```python
from build123d import *
from build123d.topology import SkipClean

# Parameters (mm, degrees)
BOSS_EXTRUDE1_START = 92.075
SKETCH1_R           = 139.7
BOSS_EXTRUDE1_DEPTH = 6.35
BOSS_EXTRUDE2_START = -92.075
SKETCH2_R           = 139.7
BOSS_EXTRUDE2_DEPTH = 12.7
BOSS_EXTRUDE3_START = 165.1
BOSS_EXTRUDE3_DEPTH = 165.1
CIRPATTERN1_COUNT   = 6
SKETCH8_R           = 38.1
BOSS_EXTRUDE4_DEPTH = 63.5
SKETCH9_R           = 19.05
CUT_EXTRUDE1_DEPTH  = 76.2
SKETCH10_R          = 101.6
CUT_EXTRUDE2_DEPTH  = 6.35


with BuildPart() as part:
    # Sketch1 → Boss-Extrude1 (new body)
    with BuildSketch(Plane(origin=(0, 0, 0), x_dir=(1, 0, 0), z_dir=(0, 1, 0)).offset(BOSS_EXTRUDE1_START)):
        with Locations(Location((0, 0, 0), (0, 0, 270))):
            Circle(SKETCH1_R)
    extrude(amount=-BOSS_EXTRUDE1_DEPTH)



with BuildPart() as body_2:
    # Sketch2 → Boss-Extrude2 (new body)
    with BuildSketch(Plane(origin=(0, 0, 0), x_dir=(1, 0, 0), z_dir=(0, 1, 0)).offset(BOSS_EXTRUDE2_START)):
        with Locations(Location((0, 0, 0), (0, 0, 270))):
            Circle(SKETCH2_R)
    extrude(amount=BOSS_EXTRUDE2_DEPTH)


with BuildPart() as part_1:
    add(part.part)

    add(body_2.part)  # Boss-Extrude3 merges body 2
    # Sketch3 → Boss-Extrude3 (add)
    with BuildSketch(Plane(origin=(0, -79.375, 0), x_dir=(1, 0, 0), z_dir=(0, 1, 0)).offset(BOSS_EXTRUDE3_START)):
        with BuildLine():
            Line((122.269799969, -59.297454545), (125.697925202, -60.96))
            ThreePointArc((125.697925202, -60.96), (135.408353278, -34.360847815), (139.555607197, -6.35))
            Line((139.555607197, -6.35), (139.555607197, 0))
            Line((139.555607197, 0), (76.563607197, 0))
            Line((76.563607197, 0), (76.563607197, -6.35))
            Line((76.563607197, -6.35), (135.741554433, -6.35))
            ThreePointArc((135.741554433, -6.35), (131.694050685, -33.507747077), (122.269799969, -59.297454545))
        make_face()
    boss_extrude3 = extrude(amount=-BOSS_EXTRUDE3_DEPTH)

    # CirPattern1: Boss-Extrude3 ×6 about axis
    with SkipClean():  # the faces are left unmerged after this step: merging them gives an invalid solid
        cirpattern1_axis = Axis((0, 0, 0), (0, 1, 0))
        for i in range(1, CIRPATTERN1_COUNT):
            add(boss_extrude3.rotate(cirpattern1_axis, i * 360 / CIRPATTERN1_COUNT))

    # Sketch8 → Boss-Extrude4 (add)
    with SkipClean():  # the faces are left unmerged after this step: merging them gives an invalid solid
        with BuildSketch(Plane.XZ.offset(92.075)):
            with Locations(Location((0, 0, 0), (0, 0, 270))):
                Circle(SKETCH8_R)
        extrude(amount=BOSS_EXTRUDE4_DEPTH)

    # Sketch9 → Cut-Extrude1 (cut)
    with SkipClean():  # the faces are left unmerged after this step: merging them gives an invalid solid
        with BuildSketch(Plane.XZ.offset(155.575)):
            with Locations(Location((0, 0, 0), (0, 0, 270))):
                Circle(SKETCH9_R)
        extrude(amount=-CUT_EXTRUDE1_DEPTH, mode=Mode.SUBTRACT)

    # Sketch10 → Cut-Extrude2 (cut)
    with SkipClean():  # the faces are left unmerged after this step: merging them gives an invalid solid
        with BuildSketch(Plane(origin=(0, 92.075, 0), x_dir=(1, 0, 0), z_dir=(0, 1, 0))):
            with Locations(Location((0, 0, 0), (0, 0, 270))):
                Circle(SKETCH10_R)
        extrude(amount=-CUT_EXTRUDE2_DEPTH, mode=Mode.SUBTRACT)


solid = part_1.part
```
Design review of the part built by this model. Coordinates are the model's own, in mm. A direction names the side the tool comes from. Give positions to 0.01 mm unless a question says otherwise; leave off trailing zeros. Loops run counter-clockwise (first coordinate to the right, second up) from the corner with the lowest first, then second, coordinate; pieces in that order, holes last. Notation, with made-up numbers: (-15.75, -2.5) -> (20.25, -2.5) arc R29 ccw to (20.25, 35.5) -> close; hole circle Ø2 at (55.5, 20.5). An arc over 180 degrees is marked (long way). One line per item, written item: value.
Q1. For L1, parallel to X at y = 88.75, z = 0; L2, parallel to Z at x = -45.5, y = -71, list the stretches that pass through material, from the lowest coordinate up.
Numbers:
L1: x = -139.7 to -101.6, 101.6 to 139.7
L2: z = -132.08 to -128.05, -91.51 to -78.81, 66.11 to 78.81
Q2. Draft analysis for pull direction Z (two halves, no side actions). For faces 4 (the flat face through (-103, 92.075, 10)), 5 (the flat face through (-109, 4, 0)), state which applies: pulls with the +Z half, pulls with the -Z half, needs draft (parallel to the pull), parting line crosses it, or undercut.
Numbers:
face 4: needs draft
face 5: undercut
Q3. Machinability: for faces 1 (the flat face through (-5, 85.725, 113)), 2 (the cylindrical face through (-131.79, 4.33, -33.13)), 3 (the flat face through (106, 4, 6.35)), which of the approach directions +Z, -Z, +X, -X, +Y, -Y give a long, thin tool a straight path to every point of the face, cutting with its end or side? Answer none if there is none.
Numbers:
face 1: none
face 2: +X
face 3: -X
Q4. We need section A-A on x = 0. Give the boundary of the cut face in (y, z) (3 decimals).
Numbers:
outline: (-155.575, -38.1) -> (-92.075, -38.1) -> (-92.075, -139.7) -> (-79.375, -139.7) -> (-79.375, -19.05) -> (-155.575, -19.05) -> close; (-155.575, 19.05) -> (-79.375, 19.05) -> (-79.375, 139.7) -> (-92.075, 139.7) -> (-92.075, 38.1) -> (-155.575, 38.1) -> close; (85.725, -139.7) -> (92.075, -139.7) -> (92.075, -101.6) -> (85.725, -101.6) -> close; (85.725, 101.6) -> (92.075, 101.6) -> (92.075, 139.7) -> (85.725, 139.7) -> close
Q5. We need section D-D on y = -97.5. Give the boundary of the cut face in (x, z).
Numbers:
outline: circle Ø76.2 at (0, 0); hole circle Ø38.1 at (0, 0)
Q6. For pin 1 Ø8 at (x, y) = (12, 24) entering from -Z; pin 2 Ø7 at (y, z) = (-22.5, 4) entering from -X; pin 3 Ø1.9 at (y, z) = (-28.5, -3) entering from +X, all flat-tipped, find the tip position at first contact; note any pin that passes through.
Numbers:
pin 1: stops at z = 134.94
pin 2: stops at x = 76.56
pin 3: stops at x = -76.56
Q7. We need section B-B on z = 11.5. Give the boundary of the cut face in (x, y) (3 decimals), and give its area (3 significant figures).
Numbers:
outline: (-139.226, -92.075) -> (-36.323, -92.075) -> (-36.323, -155.575) -> (-15.187, -155.575) -> (-15.187, -79.375) -> (-139.226, -79.375) -> close; (-139.226, 85.725) -> (-100.947, 85.725) -> (-100.947, 92.075) -> (-139.226, 92.075) -> close; (15.187, -155.575) -> (36.323, -155.575) -> (36.323, -92.075) -> (139.226, -92.075) -> (139.226, 92.075) -> (100.947, 92.075) -> (100.947, 85.725) -> (135.403, 85.725) -> (135.403, -79.375) -> (15.187, -79.375) -> close
area: 6,950 mm^2
Q8. We need section C-C on z = 106.5. Give the boundary of the cut face in (x, y) (3 decimals), and give its area (3 significant figures).
Numbers:
outline: (-90.409, -92.075) -> (90.409, -92.075) -> (90.409, -79.375) -> (61.488, -79.375) -> (61.488, 85.725) -> (90.409, 85.725) -> (90.409, 92.075) -> (-90.409, 92.075) -> close; hole (-84.403, -79.375) -> (-68.82, -79.375) -> (-68.82, 85.725) -> (-84.403, 85.725) -> close; hole (-61.488, -79.375) -> (54.155, -79.375) -> (54.155, 85.725) -> (-61.488, 85.725) -> close
area: 6,860 mm^2
